from build123d import *

# Parameters (mm, degrees)
SKETCH1_W               = 30
SKETCH1_H               = 15
BOSS_EXTRUDE1_DEPTH     = 10
CUT_EXTRUDE1_DEPTH      = 24.452078799
CUT_EXTRUDE1_DEPTH_BACK = 24.452078799
SKETCH2_W               = 7
SKETCH2_H               = 5
SKETCH3_W               = 7
SKETCH3_H               = 5
BOSS_EXTRUDE2_DEPTH     = 5


with BuildPart() as part:
    # Sketch1 → Boss-Extrude1 (new body)
    with BuildSketch(Plane(origin=(0, 0, 0), x_dir=(1, 0, 0), z_dir=(0, 1, 0))):
        Rectangle(SKETCH1_W, SKETCH1_H)
        with BuildLine():
            Line((-11, 2.75), (4, 2.75))
            ThreePointArc((4, 2.75), (6.75, 0), (4, -2.75))
            Line((4, -2.75), (-11, -2.75))
            ThreePointArc((-11, -2.75), (-13.75, 0), (-11, 2.75))
        make_face(mode=Mode.SUBTRACT)
    extrude(amount=BOSS_EXTRUDE1_DEPTH)

    # Sketch2 → Cut-Extrude1 (cut, two sides: drawn at the far end of the back side and taken through both)
    with BuildSketch(Plane.XY.offset(7.5).offset(-CUT_EXTRUDE1_DEPTH_BACK)):
        with Locations((11.5, 7.5)):
            Rectangle(SKETCH2_W, SKETCH2_H)
    extrude(amount=CUT_EXTRUDE1_DEPTH + CUT_EXTRUDE1_DEPTH_BACK, mode=Mode.SUBTRACT)

    # Sketch3 → Boss-Extrude2 (add)
    with BuildSketch(Plane(origin=(0, 5, 0), x_dir=(1, 0, 0), z_dir=(0, 1, 0))):
        with Locations((11.5, 5)):
            Rectangle(SKETCH3_W, SKETCH3_H)
    extrude(amount=BOSS_EXTRUDE2_DEPTH)


solid = part.part
Geometry check sheet. Reference: the model listing, model coordinates, mm. A direction names the side the tool comes from. Give positions to 0.01 mm unless a question says otherwise; leave off trailing zeros. Loops run counter-clockwise (first coordinate to the right, second up) from the corner with the lowest first, then second, coordinate; pieces in that order, holes last. Notation, with made-up numbers: M -40,52 L -29,52 A17 ccw -29,77 Z; hole C 59,86.5 d11. An arc over 180 degrees is marked long. Answer as a JSON object with one key per item and string values. Group by question number.
Item 1: Gauge pin test, flat ends, axial feed: pin 1 (5.5 mm diameter, centred on x = 10, z = 3.5, fed in from +Y); pin 2 (4 mm diameter, centred on y = 7.5, z = 0, fed in from +X); pin 3 (1.5 mm diameter, centred on x = 13, y = 6.5, fed in from +Z). Record the tip position at first contact, or that the pin passes through.
Item 2: Material ranges on L1, parallel to Z at x = -8.5, y = 8.25; L2, parallel to X at y = 4.25, z = -0.25, recorded low to high.
Item 3: Sectioned sample at B-B on y = 8. Record the boundary of the cut face in (x, z), plus the area to 3 significant figures.
Item 4: Sectioned sample at A-A on x = 2. Record the boundary of the cut face in (y, z).
Item 5: Sectioned sample at D-D on x = 9.75. Record the boundary of the cut face in (y, z), plus the area to 3 significant figures.
Item 6: Sectioned sample at C-C on z = 0. Record the boundary of the cut face in (x, y), plus the area to 3 significant figures.
Item 7: Mould release check, pull along Z, two halves, no side actions. Record for faces 4 (the flat face through (0, 5, 7.5)), 5 (the flat face through (11, 5, 2)), 6 (the cylindrical face through (-13.75, 4.93, 0.06)): pulls with the +Z half, pulls with the -Z half, needs draft (parallel to the pull), parting line crosses it, or undercut.
Item 8: Access from +Z, -Z, +X, -X, +Y, -Y to the whole of each face (thin tool, end or side, straight path). Record for faces 1 (the flat face through (0, 0, -3)), 2 (the flat face through (8, 7, 2)), 3 (the flat face through (-4, 5, -2.75)).
Findings below:
{
 "1": {"pin 1": "y = 10", "pin 2": "x = 8", "pin 3": "z = -2.5"},
 "2": {"L1": "-7.5 to -2.75, 2.75 to 7.5", "L2": "-15 to -13.74, 6.74 to 15"},
 "3": {"outline": "M -15,-7.5 L 15,-7.5 L 15,-2.5 L 8,-2.5 L 8,7.5 L -15,7.5 Z; hole M -11,-2.75 L 4,-2.75 A2.75 ccw 4,2.75 L -11,2.75 A2.75 ccw Z", "area": "274 mm2"},
 "4": {"outline": "M 0,-7.5 L 10,-7.5 L 10,-2.75 L 0,-2.75 Z; M 0,2.75 L 10,2.75 L 10,7.5 L 0,7.5 Z"},
 "5": {"outline": "M 0,-7.5 L 10,-7.5 L 10,-2.5 L 5,-2.5 L 5,7.5 L 0,7.5 Z", "area": "100 mm2"},
 "6": {"outline": "M -15,0 L -13.75,0 L -13.75,10 L -15,10 Z; M 6.75,0 L 15,0 L 15,5 L 8,5 L 8,10 L 6.75,10 Z", "area": "60.0 mm2"},
 "7": {"face 4": "pulls with the +Z half", "face 5": "needs draft", "face 6": "undercut"},
 "8": {"face 1": "+Z, -Z, +X, -X, -Y", "face 2": "+Z, +X, +Y", "face 3": "+Y, -Y"}
}
